Input: part model. Units: mm. Frame: model coordinates. Face numbers are marked on the shaded views. A direction names the side the tool comes from. Coordinates: 2 decimals unless noted, no trailing zeros. Loops run counter-clockwise (first coordinate to the right, second up) from the corner with the lowest first, then second, coordinate; pieces in that order, holes last. Notation, with made-up numbers: M 27.5,32 L 53.5,32 A25 cw 53.5,51 Z; hole C 54.25,61.5 d3. An arc over 180 degrees is marked long. Use a Markdown table: item, result. Add a question column.
1. Section C-C on z = 29. Output: boundary loops of the cut face in (x, y), then the cut area to 3 significant figures.
2. Section D-D on z = 11.5. Output: boundary loops of the cut face in (x, y).
3. Set-up query: the marked faces 4, 5, 6 and 7. Return all of +Z, -Z, +X, -X, +Y, -Y with unobstructed straight access to the full face (end or side cutting, diameter ignored); none if empty.
4. Pin query (flat end, axial travel): pin 1 (3 mm diameter, centred on y = 9, z = 2, fed in from -X); pin 2 (1 mm diameter, centred on x = 15.5, z = 20, fed in from -Y); pin 3 (0.8 mm diameter, centred on x = 7, z = 35.5, fed in from -Y); pin 4 (2 mm diameter, centred on x = 20, z = 22, fed in from -Y). Return the tip coordinate at first contact, or that it passes through.
5. Section A-A on y = 22.2. Output: boundary loops of the cut face in (x, z).
6. Section B-B on y = 15.5. Output: boundary loops of the cut face in (x, z).
7. Draft query along Z for the marked faces 1, 2 and 3. Return one class per face: +Z half, -Z half, draft (parallel to the pull), parting line (faces both ways), or undercut.
8. Line query: L1, parallel to Y at x = 23.25, z = 0.7; L2, parallel to X at y = 31, z = 22; L3, parallel to Y at x = 23.25, z = 36.35. Output: solid intervals per line, ascending. Write a range as [from, to].
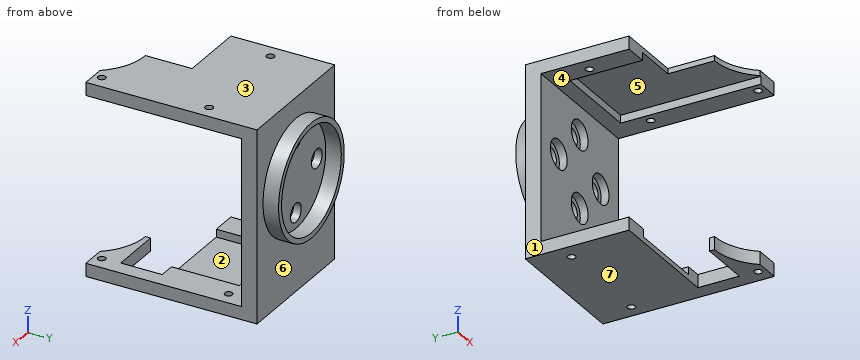
```python
from build123d import *

# Parameters (mm, degrees)
SKETCH_1_W                      = 26
SKETCH_1_H                      = 33
EXTRUDE_1_DEPTH                 = 37
SKETCH_3_W                      = 26
SKETCH_3_H                      = 32
CUT_EXTRUDE_1_DEPTH             = 30
CUT_EXTRUDE_2_REACH             = 57.982
SKETCH_2_R                      = 0.75
CUT_EXTRUDE_2_DIRECTION_2_DEPTH = 56.982140009
CUT_EXTRUDE_3_REACH             = 57.982
SKETCH_4_R                      = 0.75
SKETCH_5_W                      = 17
SKETCH_5_H                      = 1.5
CUT_EXTRUDE_4_DEPTH             = 27
CUT_EXTRUDE_5_REACH             = 57.982
SKETCH_6_W                      = 20
SKETCH_6_H                      = 8
CUT_EXTRUDE_START               = -37
CUT_EXTRUDE_6_OUTLINE_R         = 0.75
CUT_EXTRUDE_6_DEPTH             = 37
SKETCH_8_W                      = 15
SKETCH_8_H                      = 1.5
CUT_EXTRUDE_7_DEPTH             = 13
SKETCH_9_R                      = 11
SKETCH_9_R_2                    = 10
EXTRUDE_2_DEPTH                 = 3
CUT_EXTRUDE_8_REACH             = 57.982
SKETCH_10_R                     = 1.8
SKETCH_11_R                     = 2.8
CUT_EXTRUDE_9_DEPTH             = 1.5


# Read off the part's stored shape, not the designer's step: 切除-拉伸6
with BuildPart() as part:
    # 草图1 → 凸台-拉伸1 (new body)
    with BuildSketch(Plane.XY):
        with Locations((13, 16.5)):
            Rectangle(SKETCH_1_W, SKETCH_1_H)
    extrude(amount=EXTRUDE_1_DEPTH)

    # 草图3 → 切除-拉伸1 (cut)
    with BuildSketch(Plane.XZ):
        with Locations((13, 18.5)):
            Rectangle(SKETCH_3_W, SKETCH_3_H)
    extrude(amount=-CUT_EXTRUDE_1_DEPTH, mode=Mode.SUBTRACT)

    # 草图2 → 切除-拉伸2 (cut, up to next)
    with BuildSketch(Plane.XY.offset(37), mode=Mode.PRIVATE) as cut_extrude_2_sk1:
        with Locations(Location((2.75, 1.5, 0), (0, 0, 180))):
            Circle(SKETCH_2_R)
    cut_extrude_2_tool1 = extrude(cut_extrude_2_sk1.sketch, amount=-CUT_EXTRUDE_2_REACH, mode=Mode.PRIVATE) & part.part
    # 草图2 → 切除-拉伸2 (cut, up to next)
    with BuildSketch(Plane.XY.offset(37), mode=Mode.PRIVATE) as cut_extrude_2_sk2:
        with Locations(Location((23.25, 1.5, 0), (0, 0, 180))):
            Circle(SKETCH_2_R)
    cut_extrude_2_tool2 = extrude(cut_extrude_2_sk2.sketch, amount=-CUT_EXTRUDE_2_REACH, mode=Mode.PRIVATE) & part.part
    # 草图2 → 切除-拉伸2 (cut, up to next)
    with BuildSketch(Plane.XY.offset(37), mode=Mode.PRIVATE) as cut_extrude_2_sk3:
        with Locations(Location((23.25, 22.2, 0), (0, 0, 180))):
            Circle(SKETCH_2_R)
    cut_extrude_2_tool3 = extrude(cut_extrude_2_sk3.sketch, amount=-CUT_EXTRUDE_2_REACH, mode=Mode.PRIVATE) & part.part
    # 草图2 → 切除-拉伸2 (cut, up to next)
    with BuildSketch(Plane.XY.offset(37), mode=Mode.PRIVATE) as cut_extrude_2_sk4:
        with Locations(Location((2.75, 22.2, 0), (0, 0, 180))):
            Circle(SKETCH_2_R)
    cut_extrude_2_tool4 = extrude(cut_extrude_2_sk4.sketch, amount=-CUT_EXTRUDE_2_REACH, mode=Mode.PRIVATE) & part.part
    add(cut_extrude_2_tool1.solids().sort_by_distance((2.75, 1.5, 37))[0], mode=Mode.SUBTRACT)
    add(cut_extrude_2_tool2.solids().sort_by_distance((23.25, 1.5, 37))[0], mode=Mode.SUBTRACT)
    add(cut_extrude_2_tool3.solids().sort_by_distance((23.25, 22.2, 37))[0], mode=Mode.SUBTRACT)
    add(cut_extrude_2_tool4.solids().sort_by_distance((2.75, 22.2, 37))[0], mode=Mode.SUBTRACT)

    # 草图2 → 切除-拉伸2 direction 2 (cut)
    with BuildSketch(Plane.XY.offset(37)):
        with Locations(Location((2.75, 1.5, 0), (0, 0, 180))):
            Circle(SKETCH_2_R)
        with Locations(Location((23.25, 1.5, 0), (0, 0, 180))):
            Circle(SKETCH_2_R)
        with Locations(Location((23.25, 22.2, 0), (0, 0, 180))):
            Circle(SKETCH_2_R)
        with Locations(Location((2.75, 22.2, 0), (0, 0, 180))):
            Circle(SKETCH_2_R)
    extrude(amount=CUT_EXTRUDE_2_DIRECTION_2_DEPTH, mode=Mode.SUBTRACT)

    # 草图4 → 切除-拉伸3 (cut, up to next)
    with BuildSketch(Plane(origin=(0, 0, 0), x_dir=(-1, 0, 0), z_dir=(0, 0, -1)), mode=Mode.PRIVATE) as cut_extrude_3_sk1:
        with Locations((-2.75, 1.5)):
            Circle(SKETCH_4_R)
    cut_extrude_3_tool1 = extrude(cut_extrude_3_sk1.sketch, amount=-CUT_EXTRUDE_3_REACH, mode=Mode.PRIVATE) & part.part
    # 草图4 → 切除-拉伸3 (cut, up to next)
    with BuildSketch(Plane(origin=(0, 0, 0), x_dir=(-1, 0, 0), z_dir=(0, 0, -1)), mode=Mode.PRIVATE) as cut_extrude_3_sk2:
        with Locations((-23.25, 1.5)):
            Circle(SKETCH_4_R)
    cut_extrude_3_tool2 = extrude(cut_extrude_3_sk2.sketch, amount=-CUT_EXTRUDE_3_REACH, mode=Mode.PRIVATE) & part.part
    # 草图4 → 切除-拉伸3 (cut, up to next)
    with BuildSketch(Plane(origin=(0, 0, 0), x_dir=(-1, 0, 0), z_dir=(0, 0, -1)), mode=Mode.PRIVATE) as cut_extrude_3_sk3:
        with Locations((-23.25, 25.95)):
            Circle(SKETCH_4_R)
    cut_extrude_3_tool3 = extrude(cut_extrude_3_sk3.sketch, amount=-CUT_EXTRUDE_3_REACH, mode=Mode.PRIVATE) & part.part
    # 草图4 → 切除-拉伸3 (cut, up to next)
    with BuildSketch(Plane(origin=(0, 0, 0), x_dir=(-1, 0, 0), z_dir=(0, 0, -1)), mode=Mode.PRIVATE) as cut_extrude_3_sk4:
        with Locations((-3.25, 25.95)):
            Circle(SKETCH_4_R)
    cut_extrude_3_tool4 = extrude(cut_extrude_3_sk4.sketch, amount=-CUT_EXTRUDE_3_REACH, mode=Mode.PRIVATE) & part.part
    add(cut_extrude_3_tool1.solids().sort_by_distance((2.75, 1.5, 0))[0], mode=Mode.SUBTRACT)
    add(cut_extrude_3_tool2.solids().sort_by_distance((23.25, 1.5, 0))[0], mode=Mode.SUBTRACT)
    add(cut_extrude_3_tool3.solids().sort_by_distance((23.25, 25.95, 0))[0], mode=Mode.SUBTRACT)
    add(cut_extrude_3_tool4.solids().sort_by_distance((3.25, 25.95, 0))[0], mode=Mode.SUBTRACT)

    # 草图5 → 切除-拉伸4 (cut)
    with BuildSketch(Plane.XZ):
        with Locations((13, 35.25)):
            Rectangle(SKETCH_5_W, SKETCH_5_H)
    extrude(amount=-CUT_EXTRUDE_4_DEPTH, mode=Mode.SUBTRACT)

    # 草图6 → 切除-拉伸5 (cut, up to next)
    with BuildSketch(Plane(origin=(0, 0, 0), x_dir=(-1, 0, 0), z_dir=(0, 0, -1)), mode=Mode.PRIVATE) as cut_extrude_5_sk1:
        with Locations((-13, 9)):
            Rectangle(SKETCH_6_W, SKETCH_6_H)
    cut_extrude_5_tool1 = extrude(cut_extrude_5_sk1.sketch, amount=-CUT_EXTRUDE_5_REACH, mode=Mode.PRIVATE) & part.part
    add(cut_extrude_5_tool1.solids().sort_by_distance((13, 9, 0))[0], mode=Mode.SUBTRACT)

    # 切除-拉伸6 outline → 切除-拉伸6 (cut)
    with BuildSketch(Plane(origin=(0, 0, 0), x_dir=(-1, 0, 0), z_dir=(0, 0, -1)).offset(CUT_EXTRUDE_START)):
        with BuildLine():
            Line((0, 0), (0, 13))
            Line((0, 13), (-13, 13))
            Line((-13, 13), (-13, 4))
            ThreePointArc((-13, 4), (-17.582575695, 2.947221814), (-21.246211251, 0))
            Line((-21.246211251, 0), (0, 0))
        make_face()
        with Locations((-2.75, 1.5)):
            Circle(CUT_EXTRUDE_6_OUTLINE_R, mode=Mode.SUBTRACT)
    extrude(amount=CUT_EXTRUDE_6_DEPTH, mode=Mode.SUBTRACT)

    # 草图8 → 切除-拉伸7 (cut)
    with BuildSketch(Plane.XZ.offset(-13)):
        with Locations((12.397702636, 1.75)):
            Rectangle(SKETCH_8_W, SKETCH_8_H)
    extrude(amount=-CUT_EXTRUDE_7_DEPTH, mode=Mode.SUBTRACT)

    # 草图9 → 凸台-拉伸2 (add)
    with BuildSketch(Plane(origin=(0, 33, 0), x_dir=(1, 0, 0), z_dir=(0, 1, 0))):
        with Locations(Location((13, -22, 0), (0, 0, 90))):
            Circle(SKETCH_9_R)
        with Locations(Location((13, -22, 0), (0, 0, 270))):
            Circle(SKETCH_9_R_2, mode=Mode.SUBTRACT)
    extrude(amount=EXTRUDE_2_DEPTH)

    # 草图10 → 切除-拉伸8 (cut, up to next)
    with BuildSketch(Plane(origin=(0, 33, 0), x_dir=(1, 0, 0), z_dir=(0, 1, 0)), mode=Mode.PRIVATE) as cut_extrude_8_sk1:
        with Locations(Location((13, -15, 0), (0, 0, 270))):
            Circle(SKETCH_10_R)
    cut_extrude_8_tool1 = extrude(cut_extrude_8_sk1.sketch, amount=-CUT_EXTRUDE_8_REACH, mode=Mode.PRIVATE) & part.part
    # 草图10 → 切除-拉伸8 (cut, up to next)
    with BuildSketch(Plane(origin=(0, 33, 0), x_dir=(1, 0, 0), z_dir=(0, 1, 0)), mode=Mode.PRIVATE) as cut_extrude_8_sk2:
        with Locations(Location((20, -22, 0), (0, 0, 270))):
            Circle(SKETCH_10_R)
    cut_extrude_8_tool2 = extrude(cut_extrude_8_sk2.sketch, amount=-CUT_EXTRUDE_8_REACH, mode=Mode.PRIVATE) & part.part
    # 草图10 → 切除-拉伸8 (cut, up to next)
    with BuildSketch(Plane(origin=(0, 33, 0), x_dir=(1, 0, 0), z_dir=(0, 1, 0)), mode=Mode.PRIVATE) as cut_extrude_8_sk3:
        with Locations(Location((13, -29, 0), (0, 0, 270))):
            Circle(SKETCH_10_R)
    cut_extrude_8_tool3 = extrude(cut_extrude_8_sk3.sketch, amount=-CUT_EXTRUDE_8_REACH, mode=Mode.PRIVATE) & part.part
    # 草图10 → 切除-拉伸8 (cut, up to next)
    with BuildSketch(Plane(origin=(0, 33, 0), x_dir=(1, 0, 0), z_dir=(0, 1, 0)), mode=Mode.PRIVATE) as cut_extrude_8_sk4:
        with Locations(Location((6, -22, 0), (0, 0, 270))):
            Circle(SKETCH_10_R)
    cut_extrude_8_tool4 = extrude(cut_extrude_8_sk4.sketch, amount=-CUT_EXTRUDE_8_REACH, mode=Mode.PRIVATE) & part.part
    add(cut_extrude_8_tool1.solids().sort_by_distance((13, 33, 15))[0], mode=Mode.SUBTRACT)
    add(cut_extrude_8_tool2.solids().sort_by_distance((20, 33, 22))[0], mode=Mode.SUBTRACT)
    add(cut_extrude_8_tool3.solids().sort_by_distance((13, 33, 29))[0], mode=Mode.SUBTRACT)
    add(cut_extrude_8_tool4.solids().sort_by_distance((6, 33, 22))[0], mode=Mode.SUBTRACT)

    # 草图11 → 切除-拉伸9 (cut)
    with BuildSketch(Plane.XZ.offset(-30)):
        with Locations(Location((6, 22, 0), (0, 0, 270))):
            Circle(SKETCH_11_R)
        with Locations(Location((13, 29, 0), (0, 0, 270))):
            Circle(SKETCH_11_R)
        with Locations(Location((20, 22, 0), (0, 0, 270))):
            Circle(SKETCH_11_R)
        with Locations(Location((13, 15, 0), (0, 0, 270))):
            Circle(SKETCH_11_R)
    extrude(amount=-CUT_EXTRUDE_9_DEPTH, mode=Mode.SUBTRACT)


solid = part.part
```
Answers below:
| question | item | result |
|---|---|---|
| 1 | outline | M 0,30 L 10.2,30 L 10.2,31.5 L 11.2,31.5 L 11.2,33 L 5.86,33 L 5.86,36 L 4.51,36 L 4.51,33 L 0,33 Z; M 14.8,31.5 L 15.8,31.5 L 15.8,30 L 26,30 L 26,33 L 21.49,33 L 21.49,36 L 20.14,36 L 20.14,33 L 14.8,33 Z |
| 1 | area | 72.3 mm² |
| 2 | outline | M 0,30 L 26,30 L 26,33 L 16.28,33 L 16.28,36 L 9.72,36 L 9.72,33 L 0,33 Z |
| 3 | face 4 | +X, -X, -Y |
| 3 | face 5 | -Y |
| 3 | face 6 | +Y |
| 3 | face 7 | -Z, +X, -X, +Y, -Y |
| 4 | pin 1 | stops at x = 23 |
| 4 | pin 2 | stops at y = 30 |
| 4 | pin 3 | stops at y = 27 |
| 4 | pin 4 | passes through |
| 5 | outline | M 0,0 L 26,0 L 26,2.5 L 19.9,2.5 L 19.9,1 L 4.9,1 L 4.9,2.5 L 0,2.5 Z; M 0,34.5 L 2,34.5 L 2,37 L 0,37 Z; M 3.5,34.5 L 4.5,34.5 L 4.5,36 L 21.5,36 L 21.5,34.5 L 22.5,34.5 L 22.5,37 L 3.5,37 Z; M 24,34.5 L 26,34.5 L 26,37 L 24,37 Z |
| 6 | outline | M 0,0 L 26,0 L 26,2.5 L 19.9,2.5 L 19.9,1 L 4.9,1 L 4.9,2.5 L 0,2.5 Z; M 0,34.5 L 4.5,34.5 L 4.5,36 L 21.5,36 L 21.5,34.5 L 26,34.5 L 26,37 L 0,37 Z |
| 7 | face 1 | draft |
| 7 | face 2 | undercut |
| 7 | face 3 | +Z half |
| 8 | L1 | y = [0, 0.75], [2.25, 25.2], [26.7, 33] |
| 8 | L2 | x = [0, 3.2], [8.8, 17.2], [22.8, 26] |
| 8 | L3 | y = [0, 0.75], [2.25, 21.45], [22.95, 33] |
